Check sheet for the drawn part. Datum: minimum x, y, z corner. Units: mm. Coordinates: 2 decimals unless noted, no trailing zeros. Write each loop counter-clockwise with the first axis right and the second up, starting at its lowest first coordinate (ties: lowest second). Pieces come first, ordered by that corner, then holes. Notation, with made-up numbers: M 3,63 L 45,63 A28 ccw 45,85 Z; hole C 32.5,-2.5 d7. An arc over 180 degrees is marked long. Answer as CSV lines item,"result".
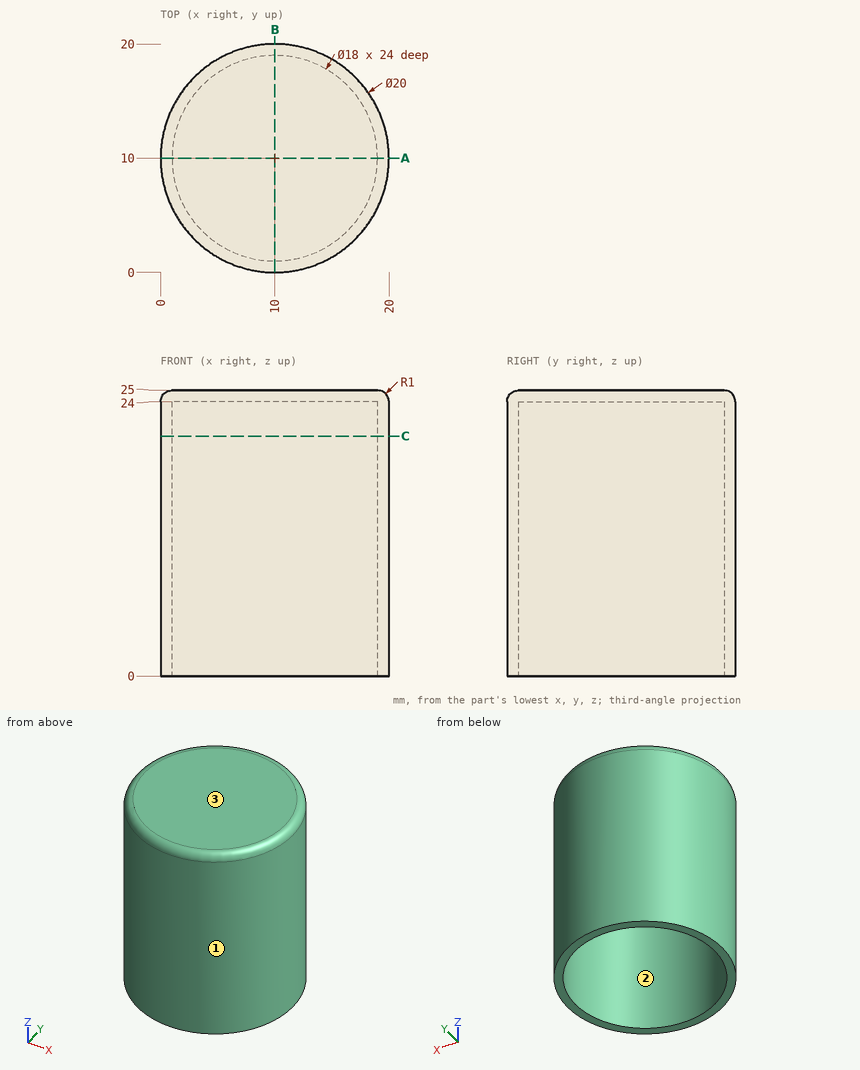
1) Thickness scan on line 1 along Y through (x, z) = (10, 19); line 2 along Z through (x, y) = (6.5, 12); line 3 along X through (y, z) = (2, 8.25). Record the ranges inside material, lowest first.
Answer key:
line 1,"y = 0 to 1, 19 to 20"
line 2,"z = 24 to 25"
line 3,"x = 4 to 5.88, 14.12 to 16"
2) Section check C-C, the plane z = 21. Record the boundary of the cut face in (x, y), plus the area to 3 significant figures.
Answer key:
outline,"C 10,10 d20; hole C 10,10 d18"
area,"59.7 mm2"
3) Section check A-A, the plane y = 10. Record the boundary of the cut face in (x, z).
Answer key:
outline,"M 0,0 L 1,0 L 1,24 L 19,24 L 19,0 L 20,0 L 20,24 A1 ccw 19,25 L 1,25 A1 ccw 0,24 Z"
4) Depth check by flat-ended pin: P1, Ø12, axis at x = 8, z = 9, coming from the -Y side; P2, Ø1.5, axis at x = 7, z = 18.5, coming from the +Y side; P3, Ø1.5, axis at y = 4.5, z = 7.5, coming from the +X side; P4, Ø5, axis at x = 3.5, z = 6.5, coming from the +Y side. Enter the tip coordinate at first touch or a pass-through.
Answer key:
P1,"stops at y = 0"
P2,"stops at y = 19.74"
P3,"stops at x = 18.8"
P4,"stops at y = 19.17"
5) Mould release check, pull along Y, two halves, no side actions. Record for the marked faces 1, 2 and 3: pulls with the +Y half, pulls with the -Y half, needs draft (parallel to the pull), parting line crosses it, or undercut.
Answer key:
face 1,"parting line crosses it"
face 2,"undercut"
face 3,"needs draft"
